Here's how the part is built. I have some questions about the finished solid (model axes, mm). Face numbers are marked on the shaded views. Give positions to 0.01 mm unless a question says otherwise; leave off trailing zeros. Loops run counter-clockwise (first coordinate to the right, second up) from the corner with the lowest first, then second, coordinate; pieces in that order, holes last. Notation, with made-up numbers: (-27.75, -33.5) - (-7.75, -33.5) arc R19 ccw to (-7.75, 1.5) - close; hole circle Ø2 at (-8.75, -6). An arc over 180 degrees is marked (long way). Return JSON: item names as keys, results as strings. Group by question number.
(1) If we mould it in two halves opening along Y, with no side actions, what happens to the marked faces 1, 2 and 3? For each: released by +Y, released by -Y, zero draft, split by the parting line, or undercut.
(2) I need wall thicknesses on probe 1 along Z at (x, y) = (15.25, 0); probe 2 along Y at (x, z) = (14.75, 0); probe 3 along Y at (x, z) = (17.5, -3). Which ranges of each line are inside material? Lowest first, please. Write a range as [from, to].
(3) If we section it at B-B (z = 0): Please give me the cut outline in (x, y).
(4) If we section it at A-A (y = 0): Please give me the cut outline in (x, z).
(5) For P1, Ø2.5, axis at x = 10.5, z = 6, coming from the +Y side; P2, Ø3, axis at x = 16.5, z = 25.5, coming from the -Y side; P3, Ø1.8, axis at x = 11.5, z = 6, coming from the -Y side, each with a flat end and sliding along its axis, tell me the tip position at first contact or that it passes through.
(6) If we section it at C-C (x = 18.5): Please give me the cut outline in (y, z), then the cut area to 3 significant figures.
```python
from build123d import *

# Parameters (mm, degrees)
SKETCH1_W          = 21
SKETCH1_H          = 32
CUT_EXTRUDE2_DEPTH = 57.382621436
CHAMFER1_SIZE      = 1


with BuildPart() as part:
    # Sketch1 → Revolve1 (revolve)
    with BuildSketch(Plane(origin=(0, 0, 0), x_dir=(1, 0, 0), z_dir=(0, 1, 0))):
        with Locations((10.5, -21)):
            Rectangle(SKETCH1_W, SKETCH1_H)
    revolve(axis=Axis((0, 0, 0), (1, 0, 0)))

    # Sketch2 → Cut-Extrude2 (cut, through all)
    with BuildSketch(Plane(origin=(0, 0, 0), x_dir=(0, 0, -1), z_dir=(1, 0, 0))):
        with BuildLine():
            Line((-4.582575695, -2), (-6.8, -2))
            Line((-6.8, -2), (-6.8, 2))
            Line((-6.8, 2), (-4.582575695, 2))
            ThreePointArc((-4.582575695, 2), (-5, 0), (-4.582575695, -2))
        make_face()
    extrude(amount=CUT_EXTRUDE2_DEPTH, mode=Mode.SUBTRACT)

    # Chamfer1
    chamfer1_edges = [part.edges().sort_by_distance(p)[0] for p in [
        (0, 0, -37),
        (21, 0, -37),
        (21, 0, -5),
        (0, 0, -5),
    ]]
    chamfer(chamfer1_edges, length=CHAMFER1_SIZE)


solid = part.part
```
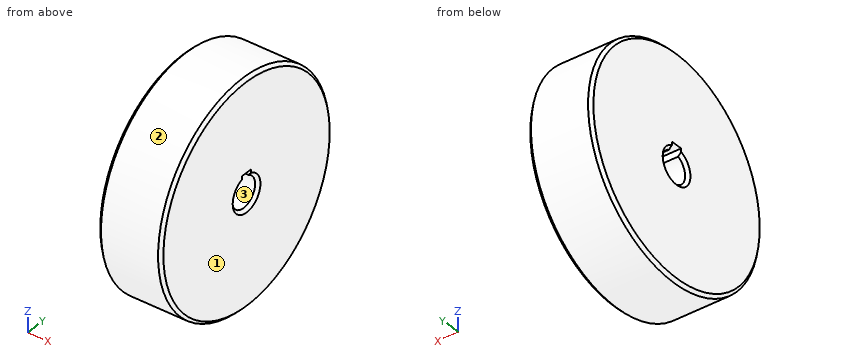
Values:
{
 "1": {"face 1": "zero draft", "face 2": "split by the parting line", "face 3": "undercut"},
 "2": {"probe 1": "[-37, -5], [6.8, 37]", "probe 2": "[-37, -5], [5, 37]", "probe 3": "[-36.88, -4], [4, 36.88]"},
 "3": {"outline": "(0, -36) - (1, -37) - (20, -37) - (21, -36) - (21, -6) - (20, -5) - (1, -5) - (0, -6) - close; (0, 6) - (1, 5) - (20, 5) - (21, 6) - (21, 36) - (20, 37) - (1, 37) - (0, 36) - close"},
 "4": {"outline": "(0, -36) - (1, -37) - (20, -37) - (21, -36) - (21, -6) - (20, -5) - (1, -5) - (0, -6) - close; (0, 6.8) - (21, 6.8) - (21, 36) - (20, 37) - (1, 37) - (0, 36) - close"},
 "5": {"P1": "y = 36.69", "P2": "y = -28.16", "P3": "y = -36.65"},
 "6": {"outline": "circle Ø74 at (0, 0); hole (-2, 4.58) arc R5 ccw (long way) to (2, 4.58) - (2, 6.8) - (-2, 6.8) - close", "area": "4,210 mm2"}
}
